Verification items for the finished model (mm, model axes). Coordinates: 2 decimals unless noted, no trailing zeros. Loops run counter-clockwise (first coordinate to the right, second up) from the corner with the lowest first, then second, coordinate; pieces in that order, holes last. Notation, with made-up numbers: (63.5, -27) -> (75.5, -27) arc R19 cw to (75.5, -19) -> close; hole circle Ø5 at (20.5, 45.25). An arc over 180 degrees is marked (long way). Use CSV: the item, a comma, the result in double quotes. Start each with the question number.
```python
from build123d import *

# Parameters (mm, degrees)
BASPROSKE_W              = 28
BASPROSKE_H              = 14
TOOTHCUT_DEPTH           = 35.292856399
TEETHCUTS_COUNT          = 12
TEETHCUTS_ANGLE          = 330
BORSKE_R                 = 5
BORE_DEPTH               = 50.0000508
KEYSKE_W                 = 4
KEYSKE_H                 = 6.8
KEYWAY_DEPTH             = 50.0000508
RESSALTO_EXTRUS_O1_START = -28
ESBO_O1_R                = 9.499
RESSALTO_EXTRUS_O1_DEPTH = 28
CORTE_EXTRUS_O1_REACH    = 35.98


with BuildPart() as part:
    # BasProSke → Base-Revolve (revolve)
    with BuildSketch(Plane(origin=(0, 0, 0), x_dir=(1, 0, 0), z_dir=(0, 1, 0)), mode=Mode.PRIVATE) as base_revolve_sk:
        with Locations((14, 7)):
            Rectangle(BASPROSKE_W, BASPROSKE_H)
    revolve(base_revolve_sk.sketch.rotate(Axis((-10, 0, 0), (1, 0, 0)), 180), axis=Axis((-10, 0, 0), (1, 0, 0)))

    # TooCutSke → ToothCut (cut, through all)
    with BuildSketch(Plane(origin=(0, 0, 0), x_dir=(0, 0, -1), z_dir=(1, 0, 0))):
        with BuildLine():
            ThreePointArc((1.111908866, 9.433698091), (0, 9.499), (-1.111908866, 9.433698091))
            ThreePointArc((-1.111908866, 9.433698091), (-1.651516138, 11.821129337), (-3.298149691, 13.632096456))
            ThreePointArc((-3.298149691, 13.632096456), (0, 14.0254), (3.298149691, 13.632096456))
            ThreePointArc((3.298149691, 13.632096456), (1.651516138, 11.821129337), (1.111908866, 9.433698091))
        make_face()
    toothcut = extrude(amount=TOOTHCUT_DEPTH, mode=Mode.SUBTRACT)

    # TeethCuts: ToothCut ×12 about axis
    teethcuts_axis = Axis((-10, 0, 0), (1, 0, 0))
    for i in range(1, TEETHCUTS_COUNT):
        add(toothcut.rotate(teethcuts_axis, i * TEETHCUTS_ANGLE / (TEETHCUTS_COUNT - 1)), mode=Mode.SUBTRACT)

    # BorSke → Bore (cut, symmetric)
    with BuildSketch(Plane(origin=(0, 0, 0), x_dir=(0, 0, -1), z_dir=(1, 0, 0))):
        with Locations(Location((0, 0, 0), (0, 0, 180))):
            Circle(BORSKE_R)
    extrude(amount=BORE_DEPTH, both=True, mode=Mode.SUBTRACT)

    # KeySke → Keyway (cut, symmetric)
    with BuildSketch(Plane(origin=(0, 0, 0), x_dir=(0, 0, -1), z_dir=(1, 0, 0))):
        with Locations((0, 3.4)):
            Rectangle(KEYSKE_W, KEYSKE_H)
    extrude(amount=KEYWAY_DEPTH, both=True, mode=Mode.SUBTRACT)

    # Esboço1 → Ressalto-extrusão1 (add)
    with BuildSketch(Plane(origin=(28, 0, 0), x_dir=(0, 0, -1), z_dir=(1, 0, 0)).offset(RESSALTO_EXTRUS_O1_START)):
        Circle(ESBO_O1_R)
    extrude(amount=RESSALTO_EXTRUS_O1_DEPTH)

    # Esboço2 → Corte-extrusão1 (cut, up to next)
    with BuildSketch(Plane(origin=(28, 0, 0), x_dir=(0, 0, -1), z_dir=(1, 0, 0)), mode=Mode.PRIVATE) as corte_extrus_o1_sk1:
        with BuildLine():
            Line((-2.85, 1.341640786), (-2.85, -1.341640786))
            ThreePointArc((-2.85, -1.341640786), (3.15, 0), (-2.85, 1.341640786))
        make_face()
    corte_extrus_o1_tool1 = extrude(corte_extrus_o1_sk1.sketch, amount=-CORTE_EXTRUS_O1_REACH, mode=Mode.PRIVATE) & part.part
    add(corte_extrus_o1_tool1.solids().sort_by_distance((28, 0, -0.052561))[0], mode=Mode.SUBTRACT)


solid = part.part
```
1. Cross-section at B-B, the plane y = 0. Record the boundary of the cut face in (x, z), plus the area to 3 significant figures.
2. Cross-section at A-A, the plane z = 0. Record the boundary of the cut face in (x, y).
3. Depth check by flat-ended pin: pin 1 (5 mm diameter, centred on y = 0, z = 0, fed in from -X); pin 2 (2 mm diameter, centred on x = 9.5, y = 0, fed in from -Z); pin 3 (1.5 mm diameter, centred on x = 5, y = 10, fed in from +Z); pin 4 (6 mm diameter, centred on x = 16.5, y = -8, fed in from -Z). Enter the tip coordinate at first touch or a pass-through.
4. Scan lines: line 1 (Y direction, x = 25.25, z = -8); line 2 (Y direction, x = 6.75, z = 9). Record each from-to range of solid material in increasing order.
5. Release check for a two-part mould opening along Z. For faces 1 (the cylindrical face through (13.8, -11.08, -4.48)), 2 (the flat face through (0, -0.2, 3.2)) record: released by +Z, released by -Z, zero draft, split by the parting line, or undercut.
6. Cross-section at C-C, the plane z = 5. Record the boundary of the cut face in (x, y), plus the area to 3 significant figures.
Solution:
1,outline,"(0, -9.5) -> (28, -9.5) -> (28, -3.15) -> (0, -3.15) -> close; (0, 2.85) -> (28, 2.85) -> (28, 9.5) -> (0, 9.5) -> close"
1,area,"364 mm2"
2,outline,"(0, -9.5) -> (28, -9.5) -> (28, -3.15) -> (0, -3.15) -> close; (0, 3.15) -> (28, 3.15) -> (28, 9.5) -> (0, 9.5) -> close"
3,pin 1,"passes through"
3,pin 2,"stops at z = -9.5"
3,pin 3,"stops at z = 10.15"
3,pin 4,"stops at z = -10.15"
4,line 1,"y = -9.76 to -5.91, -5.12 to 5.12, 5.91 to 9.76"
4,line 2,"y = -10.07 to -6.79, -3.91 to 3.91, 6.79 to 10.07"
5,face 1,"undercut"
5,face 2,"zero draft"
6,outline,"(0, -8.08) -> (28, -8.08) -> (28, 8.08) -> (0, 8.08) -> close"
6,area,"452 mm2"
